Source: three-view drawing plus pictorial views. Frame: mm from the lowest corner of the part. A direction names the side the tool comes from. Coordinates: 2 decimals unless noted, no trailing zeros. Loops run counter-clockwise (first coordinate to the right, second up) from the corner with the lowest first, then second, coordinate; pieces in that order, holes last.
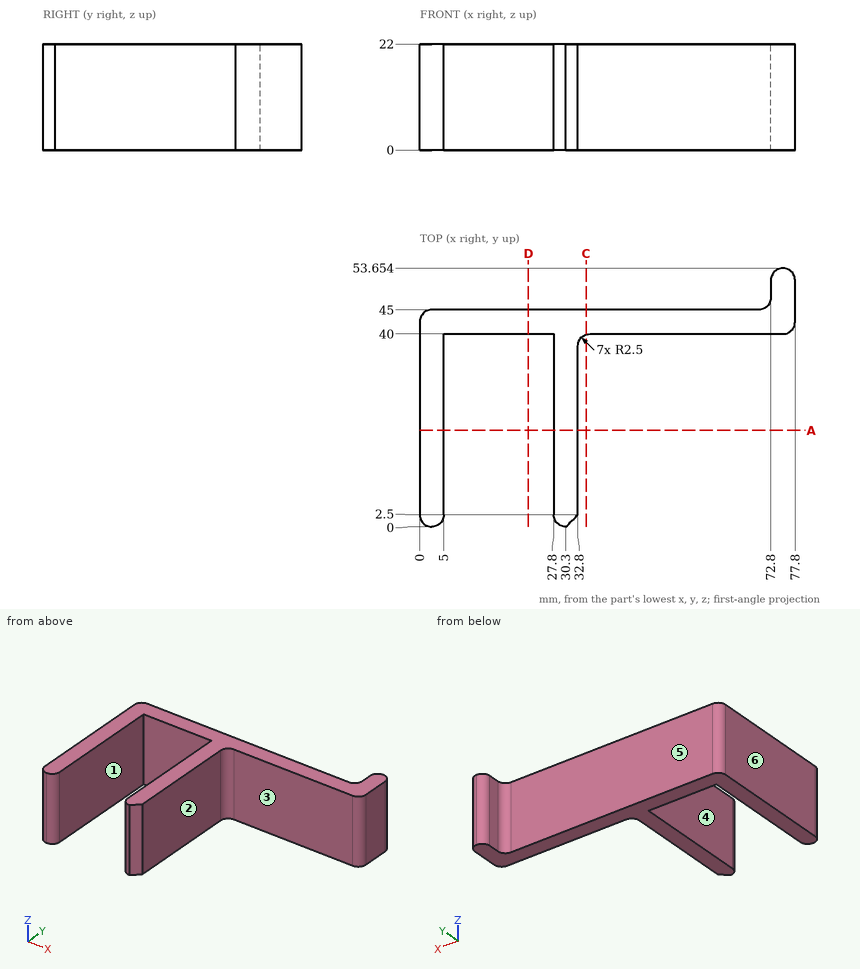
Q1. Draft query along X for the marked faces 1, 2 and 3. Return one class per face: released by +X, released by -X, zero draft, split by the parting line, or undercut.
Q2. Reachability of the marked faces 4, 5 and 6 from +Z, -Z, +X, -X, +Y, -Y: full face, straight path, thin tool, end or side. Return the list, or none.
Q3. Section query C-C on x = 34.5. Return the cut outline in (y, z).
Q4. Section query A-A on y = 20. Return the cut outline in (x, z).
Q5. Material intervals for line 1 along X through (y, z) = (24.5, 4); line 2 along Y through (x, z) = (66.5, 14.25); line 3 along X through (y, z) = (43, 3.5), sorted ascending.
Q6. First-contact query: pin 1 Ø3 at (y, z) = (37, 18.5) entering from +X; pin 2 Ø11 at (y, z) = (25.5, 9.5) entering from +X; pin 3 Ø4 at (x, z) = (10.5, 8.5) entering from -Y. Flat tips, straight axial feed; report the tip coordinate or a pass-through.
Q7. Section query D-D on x = 22.5. Return the cut outline in (y, z).
Resolved:
1. face 1: undercut
1. face 2: released by +X
1. face 3: zero draft
2. face 4: +Z, -Z, -Y
2. face 5: +Z, -Z, -X, +Y
2. face 6: +Z, -Z, -X, +Y, -Y
3. outline: (39.87, 0) - (45, 0) - (45, 22) - (39.87, 22) - close
4. outline: (0, 0) - (5, 0) - (5, 22) - (0, 22) - close; (27.8, 0) - (32.8, 0) - (32.8, 22) - (27.8, 22) - close
5. line 1: x = 0 to 5, 27.8 to 32.8
5. line 2: y = 40 to 45
5. line 3: x = 0.05 to 77.8
6. pin 1: stops at x = 33.01
6. pin 2: stops at x = 32.8
6. pin 3: stops at y = 40
7. outline: (40, 0) - (45, 0) - (45, 22) - (40, 22) - close
